Geometry check sheet. Reference: the model listing, model coordinates, mm. Face numbers are marked on the shaded views. A direction names the side the tool comes from. Round coordinates to 2 decimals unless told otherwise and drop trailing zeros. Write each loop counter-clockwise with the first axis right and the second up, starting at its lowest first coordinate (ties: lowest second). Pieces come first, ordered by that corner, then holes.
Item 1: Access from +Z, -Z, +X, -X, +Y, -Y to the whole of each face (thin tool, end or side, straight path). Record for the marked faces 1 and 2.
Item 2: Cross-section at A-A (z = 7). Enter the section's corners in (x, y).
Item 3: Depth check by flat-ended pin: P1, Ø10, axis at y = 2.5, z = 8.5, coming from the +X side; P2, Ø8, axis at x = -18, y = 3.5, coming from the +Z side. Enter the tip coordinate at first touch or a pass-through.
Item 4: Draft check along Z on the marked faces 3, 4, 5 and 6. Enter one of: pulls with the +Z half, pulls with the -Z half, needs draft (parallel to the pull), parting line crosses it, or undercut.
Item 5: Cross-section at B-B (x = -22.25). Enter the section's corners in (y, z).
Item 6: Cross-section at C-C (y = 0). Enter the section's corners in (x, z), then the cut area to 3 significant figures.
Item 7: Scan lines: probe 1 along X at (y, z) = (4.5, 15.25); probe 2 along Z at (x, y) = (-15, 3.75); probe 3 along X at (y, z) = (9.5, 5.5). Record each from-to range of solid material in increasing order.
Item 8: Cross-section at D-D (x = -26.5). Enter the section's corners in (y, z).
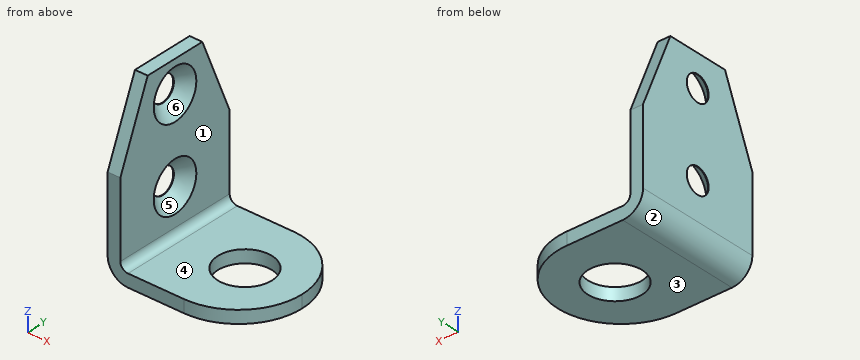
from build123d import *

# Parameters (mm, degrees)
SKETCH_1_W                       = 2
SKETCH_1_H                       = 20
SM_BASE_FLANGE_1_DEPTH           = 25
SM_EDGE_FLANGE_1_STRIP_W         = 10.4
SM_EDGE_FLANGE_1_STRIP_H         = 2
SM_EDGE_FLANGE_1_STRIP_CUT_DEPTH = 20
SM_EDGE_FLANGE_1_DEPTH           = 20
SKETCH_6_R                       = 4.25
CUT_EXTRUDE_1_DEPTH              = 10
FILLET_1_R                       = 10
SKETCH_7_R                       = 2
CUT_EXTRUDE_2_DEPTH              = 10
CUT_EXTRUDE_3_DEPTH              = 5
CHAMFER_1_SIZE                   = 1.9


# Sheet-metal steps are written as plain solids
with BuildPart() as part:
    # Sketch 1 → Базовая кромка1 (new body)
    with BuildSketch(Plane.XY):
        with Locations((-34.970714213, 7.011351052)):
            Rectangle(SKETCH_1_W, SKETCH_1_H)
    extrude(amount=SM_BASE_FLANGE_1_DEPTH)

    # Ребро-кромка1 strip (across the edge) → Ребро-кромка1 strip cut (cut)
    with BuildSketch(Plane(origin=(-33.970714213, -2.988648948, 0), x_dir=(0, 0, 1), z_dir=(0, 1, 0))):
        with Locations((-4, -1)):
            Rectangle(SM_EDGE_FLANGE_1_STRIP_W, SM_EDGE_FLANGE_1_STRIP_H)
    extrude(amount=SM_EDGE_FLANGE_1_STRIP_CUT_DEPTH, mode=Mode.SUBTRACT)

    # Ребро-кромка1 section (across the edge) → Ребро-кромка1 (add)
    with BuildSketch(Plane(origin=(-33.970714213, -2.988648948, 0), x_dir=(0, 0, 1), z_dir=(0, 1, 0))):
        with BuildLine():
            Line((-2, 1.2), (-2, 20))
            Line((-2, 20), (0, 20))
            Line((0, 20), (0, 1.2))
            ThreePointArc((0, 1.2), (0.351471863, 0.351471863), (1.2, 0))
            Line((1.2, 0), (1.2, -2))
            ThreePointArc((1.2, -2), (-1.0627417, -1.0627417), (-2, 1.2))
        make_face()
    extrude(amount=SM_EDGE_FLANGE_1_DEPTH)

    # Эскиз6 → Вырез-Вытянуть1 (cut)
    with BuildSketch(Plane.XY):
        with Locations((-22.970714213, 7.011351052)):
            Circle(SKETCH_6_R)
    extrude(amount=-CUT_EXTRUDE_1_DEPTH, mode=Mode.SUBTRACT)

    # Скругление1
    fillet_1_edges = [part.edges().sort_by_distance(p)[0] for p in [
        (-13.970714213, 17.011351052, -1),
        (-13.970714213, -2.988648948, -1),
    ]]
    fillet(fillet_1_edges, radius=FILLET_1_R - 0.0001)  # a hair under: the kernel refuses the full size

    # Эскиз7 → Вырез-Вытянуть2 (cut)
    with BuildSketch(Plane(origin=(-33.970714213, 0, 0), x_dir=(0, 0, -1), z_dir=(1, 0, 0))):
        with Locations(Location((-20, 7.011351052, 0), (0, 0, 90))):
            Circle(SKETCH_7_R)
        with Locations(Location((-7, 7.011351052, 0), (0, 0, 90))):
            Circle(SKETCH_7_R)
    extrude(amount=-CUT_EXTRUDE_2_DEPTH, mode=Mode.SUBTRACT)

    # Эскиз9 → Вырез-Вытянуть3 (cut)
    with BuildSketch(Plane(origin=(-33.970714213, 0, 0), x_dir=(0, 0, -1), z_dir=(1, 0, 0))):
        Polygon((-25, 17.011351052), (-13, 17.011351052), (-25, 12.011351052), align=None)
        Polygon((-25, 2.011351052), (-13, -2.988648948), (-25, -2.988648948), align=None)
    extrude(amount=-CUT_EXTRUDE_3_DEPTH, mode=Mode.SUBTRACT)

    # Фаска1
    chamfer_1_edges = [part.edges().sort_by_distance(p)[0] for p in [
        (-33.970714213, 5.011351052, 20),
        (-33.970714213, 5.011351052, 7),
    ]]
    chamfer(chamfer_1_edges, length=CHAMFER_1_SIZE)


solid = part.part
Resolved:
1. face 1: +Z, +X, +Y, -Y
1. face 2: -Z, -X, +Y, -Y
2. outline: (-35.97, -2.99) - (-33.97, -2.99) - (-33.97, 3.11) - (-35.87, 5.01) - (-35.97, 5.01) - close; (-35.97, 9.01) - (-35.87, 9.01) - (-33.97, 10.91) - (-33.97, 17.01) - (-35.97, 17.01) - close
3. P1: stops at x = -33.97
3. P2: stops at z = 0
4. face 3: pulls with the -Z half
4. face 4: pulls with the +Z half
4. face 5: undercut
4. face 6: undercut
5. outline: (-2.84, -2) - (2.82, -2) - (2.82, 0) - (-2.84, 0) - close; (11.2, -2) - (16.86, -2) - (16.86, 0) - (11.2, 0) - close
6. outline: (-35.97, 1.2) arc R3.2 ccw to (-32.77, -2) - (-16.84, -2) - (-16.84, 0) - (-32.77, 0) arc R1.2 cw to (-33.97, 1.2) - (-33.97, 20.17) - (-35.97, 20.17) - close
6. area: 76.7 mm2
7. probe 1: x = -35.97 to -33.97
7. probe 2: z = -2 to 0
7. probe 3: x = -35.97 to -34.96
8. outline: (-2.99, -2) - (4.64, -2) - (4.64, 0) - (-2.99, 0) - close; (9.38, -2) - (17.01, -2) - (17.01, 0) - (9.38, 0) - close
